```python
from build123d import *

# Parameters (mm, degrees)
SKETCH1_R           = 20.701
BOSS_EXTRUDE1_DEPTH = 9.525
SKETCH2_W           = 184.15
SKETCH2_H           = 63.5
SKETCH2_W_2         = 213.36
SKETCH2_H_2         = 64.479988722
CUT_EXTRUDE1_DEPTH  = 267.045158533
FILLET1_R           = 25.4
FILLET2_R           = 25.4


with BuildPart() as part:
    # Sketch1 → Boss-Extrude1 (new body)
    with BuildSketch(Plane.XY):
        Polygon((-138.259383474, 48.991487021), (32.210627804, -121.478524257), (222.710627804, -121.478524257), (222.710627804, 145.221475743), (-138.259383474, 145.221475743), align=None)
        with Locations(Location((147.490616526, 113.471475743, 0), (0, 0, 180))):
            Circle(SKETCH1_R, mode=Mode.SUBTRACT)
    extrude(amount=BOSS_EXTRUDE1_DEPTH)

    # Sketch2 → Cut-Extrude1 (cut, through all)
    with BuildSketch(Plane.XY.offset(9.525)):
        with Locations((130.635627804, -89.728524257)):
            Rectangle(SKETCH2_W, SKETCH2_H)
        with Locations((-31.579383474, 112.981481382)):
            Rectangle(SKETCH2_W_2, SKETCH2_H_2)
    extrude(amount=-CUT_EXTRUDE1_DEPTH, mode=Mode.SUBTRACT)

    # Fillet1
    fillet1_edges = [part.edges().sort_by_distance(p)[0] for p in [
        (75.100616526, 80.741487021, 4.7625),
    ]]
    fillet(fillet1_edges, radius=FILLET1_R)

    # Fillet2
    fillet2_edges = [part.edges().sort_by_distance(p)[0] for p in [
        (38.560627804, -57.978524257, 4.7625),
        (-138.259383474, 80.741487021, 4.7625),
    ]]
    fillet(fillet2_edges, radius=FILLET2_R)


solid = part.part
```
Source: CAD feature listing. Evaluate the final solid. Frame: model axes, mm. A direction names the side the tool comes from. Coordinates: 2 decimals unless noted, no trailing zeros. Write each loop counter-clockwise with the first axis right and the second up, starting at its lowest first coordinate (ties: lowest second). Pieces come first, ordered by that corner, then holes. Notation, with made-up numbers: (29, 18) -> (60, 18) arc R28 ccw to (60, 42) -> close; hole circle Ø7 at (45, 54). An arc over 180 degrees is marked (long way). Return JSON: item names as keys, results as strings. Group by question number.
1) Section query D-D, the plane x = -46. Return loops of the section in (y, z) (3 decimals), plus the area to 3 significant figures.
2) Set-up query: faces 5 (the face through (80, 43, 0)), 6 (the face through (-33, 80.741, 5)). Return all of +Z, -Z, +X, -X, +Y, -Y with unobstructed straight access to the full face (end or side cutting, diameter ignored); none if empty.
3) Contact query for flat-ended pins moving along their axis: P1, Ø3, axis at y = 124.5, z = 5.5, coming from the -X side; P2, Ø25, axis at x = 147.49, y = 113.47, coming from the -Z side; P3, Ø1, axis at x = 66.5, z = 4.5, coming from the +Y side; P4, Ø5, axis at y = -16.5, z = 3.5, coming from the -X side. Output: stop coordinate, or through.
4) Section query A-A, the plane z = 8. Return loops of the section in (x, y), plus the area to 3 significant figures.
5) Mould query, pull axis Y, two halves, no side actions, for faces 1 (the face through (142, -57.979, 5)), 2 (the face through (150, 145.221, 5)), 3 (the face through (128.37, 121.4, 4.7)), 4 (the face through (38.561, -103, 5)). Classes: +Y half, -Y half, draft (parallel to the pull), parting line (faces both ways), or undercut.
6) Section query B-B, the plane y = 101. Return loops of the section in (x, z) (3 decimals).
7) Ray query, line 1 along Y through (x, z) = (146.5, 7.75); line 2 along X through (y, z) = (127, 7); line 3 along Y through (x, z) = (205.5, 6). Return the intervals inside material, ascending.
8) Section query C-C, the plane x = 145. Return loops of the section in (y, z) (3 decimals).
From the geometry:
{
 "1": {"outline": "(-43.268, 0) -> (80.741, 0) -> (80.741, 9.525) -> (-43.268, 9.525) -> close", "area": "1,180 mm²"},
 "2": {"face 5": "-Z, +X, -X, +Y, -Y", "face 6": "+Z, -Z, -X, +Y"},
 "3": {"P1": "x = 75.1", "P2": "through", "P3": "y = 87.54", "P4": "x = -75.27"},
 "4": {"outline": "(-138.26, 48.99) -> (32.21, -121.48) -> (38.56, -121.48) -> (38.56, -83.38) arc R25.4 cw to (63.96, -57.98) -> (222.71, -57.98) -> (222.71, 145.22) -> (75.1, 145.22) -> (75.1, 106.14) arc R25.4 cw to (49.7, 80.74) -> (-112.86, 80.74) arc R25.4 ccw to (-138.26, 55.34) -> close; hole circle Ø41.4 at (147.49, 113.47)", "area": "55,100 mm²"},
 "5": {"face 1": "-Y half", "face 2": "+Y half", "face 3": "undercut", "face 4": "draft"},
 "6": {"outline": "(74.575, 0) -> (130.968, 0) -> (130.968, 9.525) -> (74.575, 9.525) -> close; (164.013, 0) -> (222.711, 0) -> (222.711, 9.525) -> (164.013, 9.525) -> close"},
 "7": {"line 1": "-57.98 to 92.79, 134.15 to 145.22", "line 2": "75.1 to 131.82, 163.16 to 222.71", "line 3": "-57.98 to 145.22"},
 "8": {"outline": "(-57.979, 0) -> (92.921, 0) -> (92.921, 9.525) -> (-57.979, 9.525) -> close; (134.022, 0) -> (145.221, 0) -> (145.221, 9.525) -> (134.022, 9.525) -> close"}
}
